Autodesk Inventor part; units mm, degrees
ref_plane "YZ Plane" through (0, 0, 0) normal (1, 0, 0) x (0, 1, 0)
ref_plane "XZ Plane" through (0, 0, 0) normal (0, 1, 0) x (-1, 0, 0)
ref_plane "XY Plane" through (0, 0, 0) normal (0, 0, 1) x (1, 0, 0)
sketch "Sketch1" plane through (0, 0, 0) normal (0, 0, 1) x (1, 0, 0)
  circle A0 centre (0, 0) radius 152.4
  circle A1 centre (0, 0) radius 12.7
  dimension "d0" = 304.8
  dimension "d1" = 25.4
extrude "Extrusion1" add sketch "Sketch1" along normal blind 6.35
sketch "Sketch2" plane through (0, 0, 6.35) normal (0, 0, 1) x (1, 0, 0)
  point P0 (0, 0)
sketch "Sketch3" plane through (0, 0, 6.35) normal (0, 0, 1) x (1, 0, 0)
  circle A0 centre (0, 0) radius 127
  circle A1 centre (0, 0) radius 123.825
  dimension "d4" = 254
  dimension "d5" = 247.65
extrude "Extrusion2" cut sketch "Sketch3" against normal blind 1.27
sketch "Sketch4" plane through (0, 0, 0) normal (0, 0, -1) x (-1, 0, 0)
  circle A0 centre (0, 0) radius 152.4
  circle A1 centre (0, 0) radius 127
  circle A2 centre (0, 0) radius 123.825
  dimension "d8" = 254
  dimension "d9" = 247.65
extrude "Extrusion3" cut sketch "Sketch4" against normal blind 1.27 contours A1
properties part number "Plate"
Can you work these out from the model? Positions are in its coordinate system, mm. A direction names the side the tool comes from. Give positions to 0.01 mm unless a question says otherwise; leave off trailing zeros. Loops run counter-clockwise (first coordinate to the right, second up) from the corner with the lowest first, then second, coordinate; pieces in that order, holes last. Notation, with made-up numbers: (25.25, -21) - (42.25, -21) arc R13 cw to (42.25, -15) - close; hole circle Ø2 at (12, 69.25). An arc over 180 degrees is marked (long way). Return JSON: item names as keys, results as strings.
1. We'd pull the mould along X, two halves only. Please class faces 1 (the face through (26, 2, 6.35)), 2 (the face through (-28, -122, 1.27)), 3 (the face through (-120.94, 92.73, 3.13)): +X half, -X half, draft (parallel to the pull), parting line (faces both ways), or undercut.
Output values:
{"face 1": "draft", "face 2": "undercut", "face 3": "parting line"}
2. I want a section at A-A on x = 0. Please give me the cut outline in (y, z) (3 decimals).
Output values:
{"outline": "(-152.4, 0) - (-127, 0) - (-127, 1.27) - (-123.825, 1.27) - (-123.825, 0) - (-12.7, 0) - (-12.7, 6.35) - (-123.825, 6.35) - (-123.825, 5.08) - (-127, 5.08) - (-127, 6.35) - (-152.4, 6.35) - close; (12.7, 0) - (123.825, 0) - (123.825, 1.27) - (127, 1.27) - (127, 0) - (152.4, 0) - (152.4, 6.35) - (127, 6.35) - (127, 5.08) - (123.825, 5.08) - (123.825, 6.35) - (12.7, 6.35) - close"}
3. I'm going to push flat-ended pins straight in: pin 1 Ø2 at (y, z) = (-89, 3.5) entering from +X; pin 2 Ø3 at (x, z) = (99.5, 5) entering from -Y; pin 3 Ø8 at (x, y) = (-12.5, 39.5) entering from -Z. Where does each tip first touch, or does it pass through?
Output values:
{"pin 1": "stops at x = 124.43", "pin 2": "stops at y = -116.71", "pin 3": "stops at z = 0"}
4. If I drill on line 1 (Y direction, x = 0, z = 0.65) (3 decimals); line 2 (X direction, y = -18, z = 6.25); line 3 (Y direction, x = -60.5, z = 5.5), over which ranges is the centre line in solid material (lowest first)?
Output values:
{"line 1": "y = -152.4 to -127, -123.825 to -12.7, 12.7 to 123.825, 127 to 152.4", "line 2": "x = -151.33 to -125.72, -122.51 to 122.51, 125.72 to 151.33", "line 3": "y = -139.88 to -111.66, -108.04 to 108.04, 111.66 to 139.88"}
5. I want a section at C-C on x = -71. Please give me the cut outline in (y, z).
Output values:
{"outline": "(-134.85, 0) - (-105.3, 0) - (-105.3, 1.27) - (-101.45, 1.27) - (-101.45, 0) - (101.45, 0) - (101.45, 1.27) - (105.3, 1.27) - (105.3, 0) - (134.85, 0) - (134.85, 6.35) - (105.3, 6.35) - (105.3, 5.08) - (101.45, 5.08) - (101.45, 6.35) - (-101.45, 6.35) - (-101.45, 5.08) - (-105.3, 5.08) - (-105.3, 6.35) - (-134.85, 6.35) - close"}
6. For faces 4 (the face through (-26.84, -120.88, 5.72)), 5 (the face through (-2.75, 12.4, 3.13)), 6 (the face through (27.53, -123.98, 0.63)), which set-ups out of +Z, -Z, +X, -X, +Y, -Y let a thin tool reach every point of the face, with its end or its side?
Output values:
{"face 4": "+Z", "face 5": "+Z, -Z", "face 6": "-Z"}
7. I want a section at D-D on y = -60.5. Please give me the cut outline in (x, z), and give its area (3 significant figures).
Output values:
{"outline": "(-139.88, 0) - (-111.66, 0) - (-111.66, 1.27) - (-108.04, 1.27) - (-108.04, 0) - (108.04, 0) - (108.04, 1.27) - (111.66, 1.27) - (111.66, 0) - (139.88, 0) - (139.88, 6.35) - (111.66, 6.35) - (111.66, 5.08) - (108.04, 5.08) - (108.04, 6.35) - (-108.04, 6.35) - (-108.04, 5.08) - (-111.66, 5.08) - (-111.66, 6.35) - (-139.88, 6.35) - close", "area": "1,760 mm²"}
